Verification items for the finished model (mm, model axes). A direction names the side the tool comes from. Round coordinates to 2 decimals unless told otherwise and drop trailing zeros. Order: outer loops, then holes, each group sorted by start corner. A loop starts at its lowest first (then second) coordinate and runs counter-clockwise, first axis right, second up.
```python
from build123d import *

# Parameters (mm, degrees)
SKETCH1_W           = 12
SKETCH1_H           = 11
BOSS_EXTRUDE1_DEPTH = 1
SKETCH2_W           = 11
SKETCH2_H           = 11
BOSS_EXTRUDE2_DEPTH = 1
SKETCH3_R           = 2.5
BOSS_EXTRUDE3_DEPTH = 8
CHAMFER1_SIZE       = 1.2
SKETCH4_R           = 2.5
BOSS_EXTRUDE4_DEPTH = 8
CHAMFER2_SIZE       = 1.2
BOSS_EXTRUDE5_DEPTH = 1
BOSS_EXTRUDE6_DEPTH = 1


with BuildPart() as part:
    # Sketch1 → Boss-Extrude1 (new body)
    with BuildSketch(Plane(origin=(0, 0, 0), x_dir=(1, 0, 0), z_dir=(0, 1, 0))):
        with Locations((6, -5.5)):
            Rectangle(SKETCH1_W, SKETCH1_H)
    extrude(amount=BOSS_EXTRUDE1_DEPTH)

    # Sketch2 → Boss-Extrude2 (add)
    with BuildSketch(Plane.ZY):
        with Locations((5.5, -4.5)):
            Rectangle(SKETCH2_W, SKETCH2_H)
    extrude(amount=BOSS_EXTRUDE2_DEPTH)

    # Sketch3 → Boss-Extrude3 (add)
    with BuildSketch(Plane.ZY.offset(1)):
        with Locations((5.5, -4.5)):
            Circle(SKETCH3_R)
    extrude(amount=BOSS_EXTRUDE3_DEPTH)

    # Chamfer1
    chamfer1_edges = [part.edges().sort_by_distance(p)[0] for p in [
        (-9, -4.5, 3),
    ]]
    chamfer(chamfer1_edges, length=CHAMFER1_SIZE)

    # Sketch4 → Boss-Extrude4 (add)
    with BuildSketch(Plane(origin=(0, 1, 0), x_dir=(1, 0, 0), z_dir=(0, 1, 0))):
        with Locations((9.5, -5.523022779)):
            Circle(SKETCH4_R)
    extrude(amount=BOSS_EXTRUDE4_DEPTH)

    # Chamfer2
    chamfer2_edges = [part.edges().sort_by_distance(p)[0] for p in [
        (7, 9, 5.523022779),
    ]]
    chamfer(chamfer2_edges, length=CHAMFER2_SIZE)

    # Sketch5 → Boss-Extrude5 (add)
    with BuildSketch(Plane.XY.offset(11)):
        Polygon((0, -10), (12, 0), (12, 1), (-1, 1), (-1, -10), align=None)
    extrude(amount=BOSS_EXTRUDE5_DEPTH)

    # Sketch6 → Boss-Extrude6 (add)
    with BuildSketch(Plane(origin=(0, 0, 0), x_dir=(-1, 0, 0), z_dir=(0, 0, -1))):
        Polygon((-12, 0), (0, -10), (1, -10), (1, 1), (-12, 1), align=None)
    extrude(amount=BOSS_EXTRUDE6_DEPTH)


solid = part.part
```
1) Scan lines: probe 1 along Z at (x, y) = (6, -4.25); probe 2 along Y at (x, z) = (1.25, 5.75); probe 3 along Y at (x, z) = (10.25, 4.75). Record each from-to range of solid material in increasing order.
2) Sectioned sample at D-D on x = 5.5. Record the cut outline in (y, z).
3) Go/stop test with flat-tipped pins: pin 1 Ø1.5 at (y, z) = (-3, 4.5) entering from +X; pin 2 Ø4 at (x, z) = (8, 2.5) entering from +Y; pin 3 Ø1 at (x, z) = (1, 4.5) entering from -Y. Record where each tip stops, or that it passes through.
4) Sectioned sample at C-C on x = 9.5. Record the cut outline in (y, z), then the cut area to 3 significant figures.
5) Sectioned sample at B-B on z = 1.5. Record the cut outline in (x, y), then the cut area to 3 significant figures.
6) Tool access check on faces 1 (the cylindrical face through (-4.352, -3.749, 7.885)), 2 (the flat face through (6, 0, 5)), 3 (the cylindrical face through (8.958, 4.352, 7.964)). Record the directions out of +Z, -Z, +X, -X, +Y, -Y that give a thin tool (end or side, any length) a straight path to the whole face; none if there is none.
7) Sectioned sample at A-A on y = -4.5. Record the cut outline in (x, z).
Returned:
1. probe 1: z = -1 to 0, 11 to 12
1. probe 2: y = 0 to 1
1. probe 3: y = 0 to 9
2. outline: (-5.42, -1) - (1, -1) - (1, 12) - (-5.42, 12) - (-5.42, 11) - (0, 11) - (0, 0) - (-5.42, 0) - close
3. pin 1: stops at x = 0
3. pin 2: stops at y = 8.93
3. pin 3: stops at y = 0
4. outline: (-2.08, -1) - (1, -1) - (1, 3.02) - (7.8, 3.02) - (9, 4.22) - (9, 6.82) - (7.8, 8.02) - (1, 8.02) - (1, 12) - (-2.08, 12) - (-2.08, 11) - (0, 11) - (0, 0) - (-2.08, 0) - close
4. area: 55.7 mm2
5. outline: (-1, -10) - (0, -10) - (0, 0) - (12, 0) - (12, 1) - (-1, 1) - close
5. area: 23.0 mm2
6. face 1: -X
6. face 2: +X, -Y
6. face 3: +Y
7. outline: (-9, 4.2) - (-7.8, 3) - (-1, 3) - (-1, -1) - (6.6, -1) - (6.6, 0) - (0, 0) - (0, 11) - (6.6, 11) - (6.6, 12) - (-1, 12) - (-1, 8) - (-7.8, 8) - (-9, 6.8) - close
